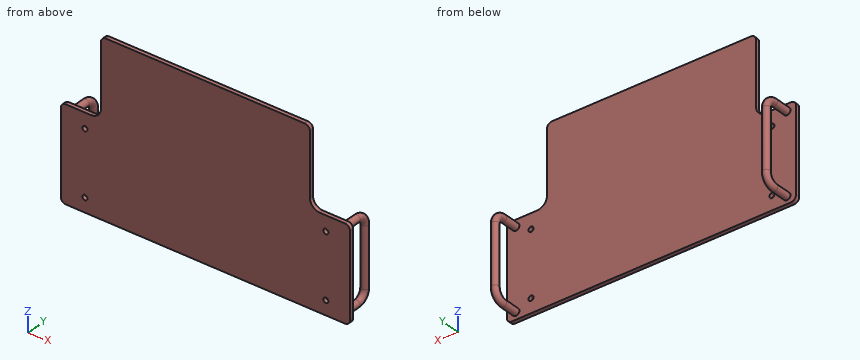
from build123d import *

# Parameters (mm, degrees)
BOSS_EXTRU_1_DEPTH      = 4
BALAYAGE13_PROFILE_R    = 3.5
BALAYAGE14_PROFILE_R    = 3.5
ESQUISSE34_R            = 2.5
ENL_V_MAT_EXTRU_1_DEPTH = 10


with BuildPart() as part:
    # Esquisse1 → Boss.-Extru.1 (new body)
    with BuildSketch(Plane(origin=(0, 0, 0), x_dir=(1, 0, 0), z_dir=(0, 1, 0))):
        with BuildLine():
            Line((5, 0), (203, 0))
            ThreePointArc((203, 0), (206.535533906, 1.464466094), (208, 5))
            Line((208, 5), (208, 67))
            ThreePointArc((208, 67), (210.928932188, 74.071067812), (218, 77))
            Line((218, 77), (243, 77))
            ThreePointArc((243, 77), (246.535533906, 78.464466094), (248, 82))
            Line((248, 82), (248, 165))
            ThreePointArc((248, 165), (246.535533906, 168.535533906), (243, 170))
            Line((243, 170), (-35, 170))
            ThreePointArc((-35, 170), (-38.535533906, 168.535533906), (-40, 165))
            Line((-40, 165), (-40, 82))
            ThreePointArc((-40, 82), (-38.535533906, 78.464466094), (-35, 77))
            Line((-35, 77), (-10, 77))
            ThreePointArc((-10, 77), (-2.928932188, 74.071067812), (0, 67))
            Line((0, 67), (0, 5))
            ThreePointArc((0, 5), (1.464466094, 1.464466094), (5, 0))
        make_face()
    extrude(amount=BOSS_EXTRU_1_DEPTH)

    # Balayage13: sweep along a path in Esquisse12
    with BuildLine(Plane(origin=(239, 0, 0), x_dir=(0, 0, -1), z_dir=(1, 0, 0))) as balayage13_path:
        Line((84, 4), (84, 20))
        ThreePointArc((84, 20), (86.928932188, 27.071067812), (94, 30))
        Line((94, 30), (153, 30))
        ThreePointArc((153, 30), (160.071067812, 27.071067812), (163, 20))
        Line((163, 20), (163, 4))
    # Balayage13 profile (on start of the path) → Balayage13 (sweep)
    with BuildSketch(Plane(origin=(239, 4, -84), x_dir=(0, 0, 1), z_dir=(0, 1, 0))):
        Circle(BALAYAGE13_PROFILE_R)
    sweep(path=balayage13_path.line)

    # Balayage14: sweep along a path in Esquisse33
    with BuildLine(Plane.ZY.offset(31)) as balayage14_path:
        Line((-163, 4), (-163, 20))
        ThreePointArc((-163, 20), (-160.071067812, 27.071067812), (-153, 30))
        Line((-153, 30), (-94, 30))
        ThreePointArc((-94, 30), (-86.928932188, 27.071067812), (-84, 20))
        Line((-84, 20), (-84, 4))
    # Balayage14 profile (on start of the path) → Balayage14 (sweep)
    with BuildSketch(Plane(origin=(-31, 4, -163), x_dir=(0, 0, 1), z_dir=(0, 1, 0))):
        Circle(BALAYAGE14_PROFILE_R)
    sweep(path=balayage14_path.line)

    # Esquisse34 → Enlèv. mat.-Extru.1 (cut)
    with BuildSketch(Plane(origin=(0, 4, 0), x_dir=(1, 0, 0), z_dir=(0, 1, 0))):
        with Locations(Location((-16, 156, 0), (0, 0, 270))):
            Circle(ESQUISSE34_R)
        with Locations(Location((224, 156, 0), (0, 0, 270))):
            Circle(ESQUISSE34_R)
        with Locations(Location((-16, 92, 0), (0, 0, 270))):
            Circle(ESQUISSE34_R)
        with Locations(Location((224, 92, 0), (0, 0, 270))):
            Circle(ESQUISSE34_R)
    extrude(amount=-ENL_V_MAT_EXTRU_1_DEPTH, mode=Mode.SUBTRACT)


solid = part.part
Geometry: final body of the model. Coordinates: model frame, mm. Give positions to 0.01 mm unless a question says otherwise; leave off trailing zeros. Write each loop counter-clockwise with the first axis right and the second up, starting at its lowest first coordinate (ties: lowest second). Pieces come first, ordered by that corner, then holes.
(1) First-contact query: P1, Ø3, axis at x = 224, z = -92, coming from the +Y side; P2, Ø4.5, axis at x = 230, y = 3, coming from the +Z side; P3, Ø2, axis at y = 2.5, z = -41, coming from the +X side; P4, Ø2, axis at y = 1.5, z = -48, coming from the -X side. Flat tips, straight axial feed; report the tip coordinate or a pass-through.
(2) Cut plane C-C, the plane y = 12. Return loops of the section in (x, z), then the cut area to 3 significant figures.
(3) Ray query, line 1 (X direction, y = 3.05, z = -92); line 2 (Z direction, x = 224, y = 1.3); line 3 (Y direction, x = 42, z = -69). Return the intervals inside material, ascending.
(4) Cut plane A-A, the plane z = -146.5. Return loops of the section in (x, y).
(5) Cut plane D-D, the plane x = 13.5. Return loops of the section in (y, z).
(6) Cut plane B-B, the plane x = -31. Return loops of the section in (y, z), then the cut area to 3 significant figures.
Values follow:
1. P1: passes through
1. P2: stops at z = -77
1. P3: stops at x = 208
1. P4: stops at x = 0
2. outline: circle Ø7 at (-31, -163); circle Ø7 at (-31, -84); circle Ø7 at (239, -163); circle Ø7 at (239, -84)
2. area: 154 mm2
3. line 1: x = -40 to -18.5, -13.5 to 221.5, 226.5 to 248
3. line 2: z = -170 to -158.5, -153.5 to -94.5, -89.5 to -77
3. line 3: y = 0 to 4
4. outline: (-40, 0) - (248, 0) - (248, 4) - (-40, 4) - close; circle Ø7 at (-31, 30); circle Ø7 at (239, 30)
5. outline: (0, -170) - (4, -170) - (4, 0) - (0, 0) - close
6. outline: (0, -170) - (4, -170) - (4, -166.5) - (20, -166.5) arc R13.5 ccw to (33.5, -153) - (33.5, -94) arc R13.5 ccw to (20, -80.5) - (4, -80.5) - (4, -77) - (0, -77) - close; hole (4, -159.5) - (20, -159.5) arc R6.5 ccw to (26.5, -153) - (26.5, -94) arc R6.5 ccw to (20, -87.5) - (4, -87.5) - close
6. area: 1,230 mm2
